Can you work these out from the drawing? Everything is in mm from the part's minimum corner. A direction names the side the tool comes from. Coordinates: 2 decimals unless noted, no trailing zeros. Order: outer loops, then holes, each group sorted by start corner. A loop starts at its lowest first (then second) coordinate and runs counter-clockwise, first axis right, second up. Notation, with made-up numbers: (-0.5, -8) -> (51.5, -8) arc R14 ccw to (51.5, -4) -> close; hole circle Ø7 at (48.25, 84). An arc over 180 degrees is marked (long way). Answer in a Markdown table with one row per item.
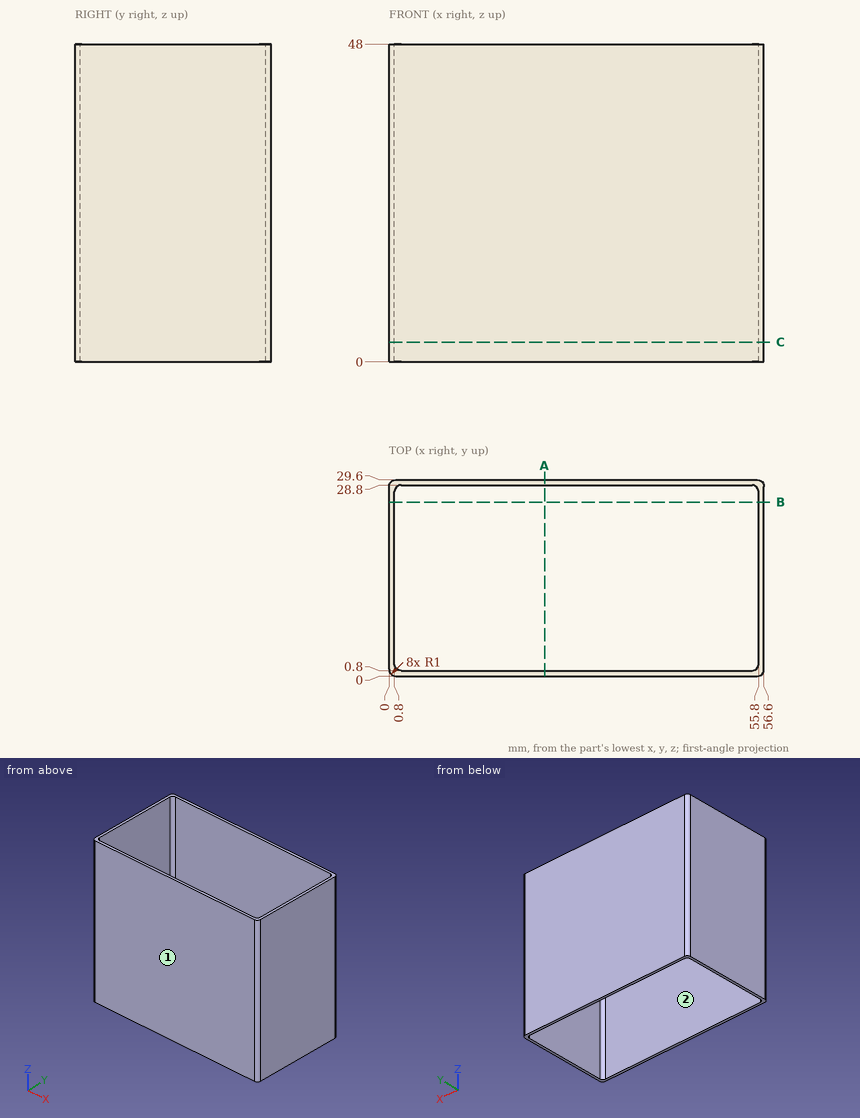
(1) On a 3-axis mill with a long thin cutter (end or side, diameter ignored), from which of +Z, -Z, +X, -X, +Y, -Y can I reach the whole of each face in a straight line? I mean the marked faces 1 and 2. Say none if no direction works.
Response values:
| item | result |
|---|---|
| face 1 | +Z, -Z, +X, -X, -Y |
| face 2 | +Z, -Z |
(2) I need wall thicknesses on line 1 (Y direction, x = 6, z = 19.5); line 2 (X direction, y = 13, z = 26). Which ranges of each line are inside material? Lowest first, please. Write a range as [from, to].
Response values:
| item | result |
|---|---|
| line 1 | [0, 0.8], [28.8, 29.6] |
| line 2 | [0, 0.8], [55.8, 56.6] |
(3) Suppose I cut it at A-A (x = 23.5). Please give me the cut outline in (y, z).
Response values:
| item | result |
|---|---|
| outline | (0, 0) -> (0.8, 0) -> (0.8, 48) -> (0, 48) -> close; (28.8, 0) -> (29.6, 0) -> (29.6, 48) -> (28.8, 48) -> close |
(4) Suppose I cut it at C-C (z = 3). Please give me the cut outline in (x, y), and give its area (3 significant figures).
Response values:
| item | result |
|---|---|
| outline | (0, 1) arc R1 ccw to (1, 0) -> (55.6, 0) arc R1 ccw to (56.6, 1) -> (56.6, 28.6) arc R1 ccw to (55.6, 29.6) -> (1, 29.6) arc R1 ccw to (0, 28.6) -> close; hole (0.8, 1.8) arc R1 ccw to (1.8, 0.8) -> (54.8, 0.8) arc R1 ccw to (55.8, 1.8) -> (55.8, 27.8) arc R1 ccw to (54.8, 28.8) -> (1.8, 28.8) arc R1 ccw to (0.8, 27.8) -> close |
| area | 135 mm2 |
(5) Suppose I cut it at B-B (y = 26.25). Please give me the cut outline in (x, z).
Response values:
| item | result |
|---|---|
| outline | (0, 0) -> (0.8, 0) -> (0.8, 48) -> (0, 48) -> close; (55.8, 0) -> (56.6, 0) -> (56.6, 48) -> (55.8, 48) -> close |
